Geometry: final body of the model. Coordinates: model frame, mm. Face numbers are marked on the shaded views. A direction names the side the tool comes from. Give positions to 0.01 mm unless a question says otherwise; leave off trailing zeros. Loops run counter-clockwise (first coordinate to the right, second up) from the corner with the lowest first, then second, coordinate; pieces in that order, holes last. Notation, with made-up numbers: (21.5, -18.5) - (80.5, -18.5) arc R36 ccw to (80.5, 19.5) - close; hole circle Ø9 at (-28, -21.75). An arc over 180 degrees is marked (long way). Use one line per item in the form item = value.
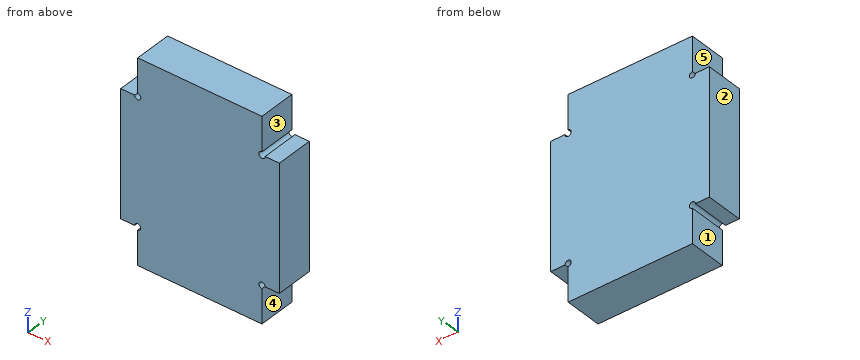
```python
from build123d import *

# Parameters (mm, degrees)
BOSS_EXTRUDE1_DEPTH = 3


with BuildPart() as part:
    # Sketch1 → Boss-Extrude1 (new body)
    with BuildSketch(Plane(origin=(0, 0, 0), x_dir=(1, 0, 0), z_dir=(0, 1, 0))):
        with BuildLine():
            Line((0.25, 5.332122905), (1.4, 5.332122905))
            Line((1.4, 5.332122905), (1.4, -4.767877095))
            Line((1.4, -4.767877095), (0.25, -4.767877095))
            ThreePointArc((0.25, -4.767877095), (-0.176776695, -4.5911004), (0, -5.017877095))
            Line((0, -5.017877095), (0, -7.767877095))
            Line((0, -7.767877095), (-10, -7.767877095))
            Line((-10, -7.767877095), (-10, -5.017877095))
            ThreePointArc((-10, -5.017877095), (-9.823223305, -4.5911004), (-10.25, -4.767877095))
            Line((-10.25, -4.767877095), (-11.364691425, -4.767877095))
            Line((-11.364691425, -4.767877095), (-11.364691425, 5.332122905))
            Line((-11.364691425, 5.332122905), (-10.245259273, 5.332122905))
            ThreePointArc((-10.245259273, 5.332122905), (-9.826575505, 5.15869841), (-10, 5.577382178))
            Line((-10, 5.577382178), (-10, 8.332122905))
            Line((-10, 8.332122905), (0, 8.332122905))
            Line((0, 8.332122905), (0, 5.582122905))
            ThreePointArc((0, 5.582122905), (-0.176776695, 5.15534621), (0.25, 5.332122905))
        make_face()
    extrude(amount=BOSS_EXTRUDE1_DEPTH)


solid = part.part
```
(1) Cut plane B-B (z = -6). Return the cut outline in (x, y).
Solution:
outline = (-10, 0) - (0, 0) - (0, 3) - (-10, 3) - close
(2) Pin query (flat end, axial travel): P1, Ø1.3, axis at x = 1, y = 1.5, coming from the +Z side; P2, Ø1.3, axis at x = 1, y = 2, coming from the -Z side; P3, Ø0.8, axis at y = 1.5, z = 7, coming from the +X side; P4, Ø4, axis at x = -9.5, z = 4, coming from the -Y side. Return the tip coordinate at first contact, or that it passes through.
Solution:
P1 = 4.77
P2 = -5.33
P3 = 0
P4 = 0
(3) Material intervals for L1, parallel to X at y = 1.6, z = -5.75; L2, parallel to Z at x = -10.75, y = 2.05; L3, parallel to X at y = 2.65, z = -5.5, sorted ascending. Write a range as from..to.
Solution:
L1 = -10..0
L2 = -5.33..4.77
L3 = -9.82..-0.19
(4) Access query for the marked faces 1, 2, 3, 4 and 5. Directions: +Z, -Z, +X, -X, +Y, -Y. A direction counts if a zero-diameter tool reaches every point of the face in a straight line with its end or side. Return the directions, or none.
Solution:
face_1 = -Z, -X, +Y, -Y
face_2 = +Z, -Z, -X, +Y, -Y
face_3 = +Z, +X, +Y, -Y
face_4 = -Z, +X, +Y, -Y
face_5 = +Z, -X, +Y, -Y
(5) Cut plane A-A (y = 2.5). Return the cut outline in (x, z).
Solution:
outline = (-11.36, -5.33) - (-10.25, -5.33) arc R0.25 cw (long way) to (-10, -5.58) - (-10, -8.33) - (0, -8.33) - (0, -5.58) arc R0.25 cw (long way) to (0.25, -5.33) - (1.4, -5.33) - (1.4, 4.77) - (0.25, 4.77) arc R0.25 cw (long way) to (0, 5.02) - (0, 7.77) - (-10, 7.77) - (-10, 5.02) arc R0.25 cw (long way) to (-10.25, 4.77) - (-11.36, 4.77) - close
